from build123d import *

# Parameters (mm, degrees)
PAD001_DEPTH    = 3.75
PAD_DEPTH       = 10
SKETCH002_W     = 1.6
SKETCH002_H     = 8.4
POCKET_DEPTH    = 7
SKETCH006_R     = 3.2
POCKET001_DEPTH = 7
SKETCH007_R     = 1.6
POCKET002_DEPTH = 8
SKETCH008_W     = 2.5
SKETCH008_H     = 7.6
POCKET003_DEPTH = 5.5
SKETCH009_W     = 3
SKETCH009_H     = 3
POCKET004_DEPTH = 12


with BuildPart() as revolution:
    # Sketch004 → Revolution (revolve)
    with BuildSketch(Plane.YZ):
        with BuildLine():
            Line((0, 24), (0, 10))
            Line((0, 10), (3.75, 10))
            Line((3.75, 10), (3.75, 13))
            ThreePointArc((3.75, 13), (3.675928, 13.53926), (3.459199, 14.038576))
            Line((3.459199, 14.038576), (2.290801, 15.961424))
            ThreePointArc((2, 17), (2.074072, 16.46074), (2.290801, 15.961424))
            Line((2, 17), (2, 24))
            Line((2, 24), (0, 24))
        make_face()
    revolve(axis=Axis((0, 0, 0), (0, 0, 1)))


with BuildPart() as pad001:
    # Sketch005 → Pad001 (new body, symmetric)
    with BuildSketch(Plane.XZ):
        with BuildLine():
            Line((-6.5, 7.1), (-6.5, 7.6))
            ThreePointArc((-6.3302, 8.157466), (-6.456609, 7.891376), (-6.5, 7.6))
            Line((-6.3302, 8.157466), (-3.75, 12))
            Line((-3.75, 12), (0, 12))
            Line((0, 12), (0, 7.1))
            Line((0, 7.1), (-6.5, 7.1))
        make_face()
    extrude(amount=PAD001_DEPTH, both=True)


with BuildPart() as pocket004:
    # Sketch → Pad (new body, symmetric)
    with BuildSketch(Plane.XZ):
        with BuildLine():
            Line((0, 0), (0, 22))
            Line((0, 22), (-3.5, 22))
            ThreePointArc((-3.5, 22), (-4.064603, 21.825362), (-4.432005, 21.362446))
            Line((-4.432005, 21.362446), (-7.932005, 12.362446))
            ThreePointArc((-7.932005, 12.362446), (-7.982854, 12.184385), (-8, 12))
            Line((-8, 12), (-8, 0))
            Line((-8, 0), (0, 0))
        make_face()
    extrude(amount=PAD_DEPTH, both=True)

    # Sketch002 → Pocket (cut)
    with BuildSketch(Plane(origin=(0, 0, 0), x_dir=(0, 0, 1), z_dir=(1, 0, 0))):
        with Locations((6.3, 0)):
            Rectangle(SKETCH002_W, SKETCH002_H)
    extrude(amount=-POCKET_DEPTH, mode=Mode.SUBTRACT)

    # Cut: cut Pad001
    add(pad001.part, mode=Mode.SUBTRACT)

    # Cut001: cut Revolution
    add(revolution.part, mode=Mode.SUBTRACT)

    # Sketch006 → Pocket001 (cut)
    with BuildSketch(Plane(origin=(-8, 0, 0), x_dir=(0, -1, 0), z_dir=(-1, 0, 0))):
        with Locations((-6, 18)):
            Circle(SKETCH006_R)
        with Locations((6, 18)):
            Circle(SKETCH006_R)
    extrude(amount=-POCKET001_DEPTH, mode=Mode.SUBTRACT)

    # Sketch007 → Pocket002 (cut)
    with BuildSketch(Plane(origin=(-8, 0, 0), x_dir=(0, -1, 0), z_dir=(-1, 0, 0))):
        with Locations((-6, 18)):
            Circle(SKETCH007_R)
        with Locations((6, 18)):
            Circle(SKETCH007_R)
    extrude(amount=-POCKET002_DEPTH, mode=Mode.SUBTRACT)

    # Sketch008 → Pocket003 (cut)
    with BuildSketch(Plane(origin=(0, 0, 0), x_dir=(1, 0, 0), z_dir=(0, 0, -1))):
        with Locations((-1.25, 0)):
            Rectangle(SKETCH008_W, SKETCH008_H)
    extrude(amount=-POCKET003_DEPTH, mode=Mode.SUBTRACT)

    # Sketch009 → Pocket004 (cut)
    with BuildSketch(Plane(origin=(0, 0, 0), x_dir=(1, 0, 0), z_dir=(0, 0, -1))):
        with Locations((-8, 6)):
            Rectangle(SKETCH009_W, SKETCH009_H)
        with Locations((-8, -6)):
            Rectangle(SKETCH009_W, SKETCH009_H)
    extrude(amount=-POCKET004_DEPTH, mode=Mode.SUBTRACT)


solid = pocket004.part
For this review, take the finished solid that the model builds, in its own axes (mm). A direction names the side the tool comes from. Coordinates: 2 decimals unless noted, no trailing zeros. Order: outer loops, then holes, each group sorted by start corner. A loop starts at its lowest first (then second) coordinate and runs counter-clockwise, first axis right, second up. Notation, with made-up numbers: (35, -3.75) - (89, -3.75) arc R22 cw to (89, 34.25) - close; hole circle Ø11 at (44.25, 75.5). An arc over 180 degrees is marked (long way). Use one line per item in the form item = value.
Q1. Consider section A-A (y = 6). Give the boundary of the cut face in (x, z), then the cut area to 3 significant figures.
Checked values:
outline = (-8, 12) - (-6.5, 12) - (-6.5, 0) - (0, 0) - (0, 16.4) - (-1, 16.4) - (-1, 14.8) - (-6.98, 14.8) - (-7.93, 12.36) arc R1 ccw to start; (-4.5, 21.2) - (-1, 21.2) - (-1, 19.6) - (0, 19.6) - (0, 22) - (-3.5, 22) arc R1 ccw to (-4.43, 21.36) - close
area = 106 mm2
Q2. Consider section C-C (z = 18.5). Give the boundary of the cut face in (x, y).
Checked values:
outline = (-5.55, -10) - (0, -10) - (0, -7.52) - (-1, -7.52) - (-1, -9.16) - (-5.55, -9.16) - close; (-5.55, -2.84) - (-1, -2.84) - (-1, -4.48) - (0, -4.48) - (0, -2) arc R2 cw to (0, 2) - (0, 4.48) - (-1, 4.48) - (-1, 2.84) - (-5.55, 2.84) - close; (-5.55, 9.16) - (-1, 9.16) - (-1, 7.52) - (0, 7.52) - (0, 10) - (-5.55, 10) - close
Q3. Draft analysis for pull direction Z (two halves, no side actions). For faces 1 (the flat face through (-2, 3.75, 10)), 2 (the flat face through (-7, -7.5, 6)), 3 (the flat face through (-4, 0, 0)), state which applies: +Z half, -Z half, draft (parallel to the pull), parting line (faces both ways), or undercut.
Checked values:
face_1 = undercut
face_2 = draft
face_3 = -Z half
Q4. Consider section D-D (z = 11.5). Give the boundary of the cut face in (x, y), then the cut area to 3 significant figures.
Checked values:
outline = (-8, -10) - (0, -10) - (0, -3.75) - (-4.09, -3.75) - (-4.09, 3.75) - (0, 3.75) - (0, 10) - (-8, 10) - (-8, 7.5) - (-6.5, 7.5) - (-6.5, 4.5) - (-8, 4.5) - (-8, -4.5) - (-6.5, -4.5) - (-6.5, -7.5) - (-8, -7.5) - close
area = 120 mm2
Q5. For probe 1 along Y at (x, z) = (-4.8, 18); probe 2 along Y at (x, z) = (-6.75, 2.75); probe 3 along Y at (x, z) = (-5.5, 6.5), list the stretches that pass through material, from the lowest coordinate up. Write a range as from..to.
Checked values:
probe_1 = -10..-9.2, -2.8..2.8, 9.2..10
probe_2 = -10..-7.5, -4.5..4.5, 7.5..10
probe_3 = -10..-4.2, 4.2..10
Q6. For faces 4 (the cylindrical face through (-3.381, 6.694, 14.876)), 5 (the flat face through (-3, 0, 22)), 6 (the flat face through (-2.5, 0, 3)), 7 (the conical face through (-2.607, 0.057, 15.441)), 8 (the flat face through (-7, 6, 12)), list the 3-axis set-ups (+Z, -Z, +X, -X, +Y, -Y) from which the entire face can be reached by the end or side of a thin tool; tool diameter is ignored.
Checked values:
face_4 = -X
face_5 = +Z, +X, -X, +Y, -Y
face_6 = -Z, +X
face_7 = +X
face_8 = -Z, -X
Q7. Consider section B-B (z = 5.75). Give the boundary of the cut face in (x, y), then the cut area to 3 significant figures.
Checked values:
outline = (-8, -10) - (0, -10) - (0, -4.2) - (-7, -4.2) - (-7, 4.2) - (0, 4.2) - (0, 10) - (-8, 10) - (-8, 7.5) - (-6.5, 7.5) - (-6.5, 4.5) - (-8, 4.5) - (-8, -4.5) - (-6.5, -4.5) - (-6.5, -7.5) - (-8, -7.5) - close
area = 92.2 mm2
Q8. For P1, Ø7.5, axis at y = -6, z = 18, coming from the -X side; P2, Ø1.2, axis at x = -7.5, y = -5.5, coming from the -Z side; P3, Ø2.5, axis at y = -6, z = 6.5, coming from the -X side, all flat-tipped, find the tip position at first contact; note any pin that passes through.
Checked values:
P1 = -7.2
P2 = 12
P3 = -6.5
